CAD build for the part. Positions are in the model's coordinates, mm. A direction names the side the tool comes from. Round coordinates to 2 decimals unless told otherwise and drop trailing zeros. Loops run counter-clockwise (first coordinate to the right, second up) from the corner with the lowest first, then second, coordinate; pieces in that order, holes last. Notation, with made-up numbers: M 42.5,30 L 78.5,30 A24 cw 78.5,59 Z; hole C 8.5,33 d5. An arc over 180 degrees is marked long. Use one line per item in the form item = value.
Autodesk Inventor part; units mm, degrees
ref_plane "Work Plane1" through (0, 0, -15) normal (0, 0, 1) x (1, 0, 0)
ref_plane "YZ Plane" through (0, 0, 0) normal (1, 0, 0) x (0, 1, 0)
ref_plane "XZ Plane" through (0, 0, 0) normal (0, 1, 0) x (-1, 0, 0)
sketch "Sketch1" plane through (0, 0, 0) normal (0, 0, 1) x (1, 0, 0)
  line L0 (0, 0) -> (25, 0)
  line L1 (25, 0) -> (25, 40)
  line L2 (25, 40) -> (0, 40)
  line L3 (0, 40) -> (0, 0)
  dimension "d1" = 25
  dimension "d2" = 40
  dimension "d3" = 25
extrude "Extrusion1" add sketch "Sketch1" against normal blind 30
sketch "Sketch2" plane through (25, 0, 0) normal (1, 0, 0) x (0, 0, -1)
  line L0 (0, 0) -> (30, 0)
  circle A0 centre (15, 6.56) radius 2.46
extrude "Extrusion2" cut sketch "Sketch2" against normal blind 30
sketch "Sketch3" plane through (0, 0, 0) normal (-1, 0, 0) x (0, 0, 1)
  line L0 (0, 0) -> (-30, 0)
  line L1 (-25.05, 0) -> (-4.95, 0)
  line L2 (-4.95, 0) -> (-4.95, 33.12)
  line L3 (-4.95, 33.12) -> (-25.05, 33.12)
  line L4 (-25.05, 33.12) -> (-25.05, 0)
  dimension "d11" = 20.1
extrude "Extrusion3" cut sketch "Sketch3" against normal blind 20
sketch "Sketch4" plane through (0, 0, 0) normal (0, -1, 0) x (1, 0, 0)
  line L0 (20, -4.95) -> (20, -25.05)
  line L1 (20, -15) -> (25, -15)
  line L2 (25, 0) -> (25, -30)
  line L3 (20, -8.025) -> (25, -8.025)
  line L4 (25, -8.025) -> (25, -21.975)
  line L5 (25, -21.975) -> (20, -21.975)
  line L6 (20, -21.975) -> (20, -8.025)
  line L7 (20, -8.025) -> (25, -21.975) construction
  line L8 (25, -8.025) -> (20, -21.975) construction
  line L9 (25, -12.54) -> (25, -17.46)
  point P0 (0, 0)
  point P1 (22.5, -15)
  dimension "d14" = 13.95
extrude "Extrusion4" add sketch "Sketch4" along normal blind 15
sketch "Sketch5" plane through (20, 0, 0) normal (-1, 0, 0) x (0, 0, 1)
  circle A0 centre (-15, 6.56) radius 2.46
  circle A1 centre (-15, 6.56) radius 4.7025
  circle A2 centre (-15, 6.56) radius 2.46
  circle A3 centre (-15, 6.56) radius 2.46
  point P0 (0, 0)
  dimension "d17" = 9.405
extrude "Extrusion5" cut sketch "Sketch5" against normal blind 2.1
sketch "Sketch6" plane through (25, 0, 0) normal (1, 0, 0) x (0, 0, -1)
  circle A0 centre (15, 6.56) radius 4.7025
  line L0 (15, 6.56) -> (15, 23.56)
  circle A1 centre (15, 23.56) radius 2.46
  point P0 (0, 0)
  dimension "d20" = 17
  dimension "d21" = 4.92
extrude "Extrusion6" cut sketch "Sketch6" against normal blind 10 contours A1
sketch "Sketch7" plane through (20, 0, 0) normal (-1, 0, 0) x (0, 0, 1)
  circle A0 centre (-15, 23.56) radius 2.46
  circle A1 centre (-15, 23.56) radius 4.7025
  point P0 (0, 0)
  dimension "d24" = 9.405
extrude "Extrusion7" cut sketch "Sketch7" against normal blind 2.1
sketch "Sketch9" plane through (25, 0, 0) normal (1, 0, 0) x (0, 0, -1)
  circle A0 centre (15, 6.56) radius 2.46
  circle A1 centre (15, 6.56) radius 2.46
  circle A2 centre (15, 23.56) radius 2.46
  circle A3 centre (15, 23.56) radius 2.46
  line L0 (30, 40) -> (30, 0)
  line L1 (30, 0) -> (30, 40)
  line L2 (30, 40) -> (0, 40)
  line L3 (0, 40) -> (0, 0)
  line L4 (0, 0) -> (8.025, 0)
  line L5 (21.975, 0) -> (21.975, -15)
  line L6 (21.975, -15) -> (8.025, -15)
  line L7 (8.025, -15) -> (8.025, 0)
  line L8 (0, 0) -> (8.025, 0)
  line L9 (21.975, 0) -> (30, 0)
extrude "Extrusion8" add sketch "Sketch9" along normal blind 5
sketch "Sketch10" plane through (0, 40, 0) normal (0, 1, 0) x (1, 0, 0)
  line L0 (0, 30) -> (30, 30)
  line L1 (30, 0) -> (0, 0)
  line L2 (0, 30) -> (30, 30)
  line L3 (30, 30) -> (30, 0)
  line L4 (30, 0) -> (0, 0)
  line L5 (0, 0) -> (0, 30)
extrude "Extrusion9" add sketch "Sketch10" along normal blind 30
sketch "Sketch12" plane through (30, 0, 0) normal (1, 0, 0) x (0, 0, -1)
  circle A0 centre (15, 6.56) radius 2.46
  line L0 (15, 6.56) -> (15, 15.06)
  circle A1 centre (15, 15.06) radius 2.525
  point P0 (0, 0)
  dimension "d31" = 8.5
  dimension "d33" = 5.05
extrude "Extrusion10" cut sketch "Sketch12" against normal blind 30 contours A1
sketch "Sketch15" plane through (0, 0, -25.05) normal (-1, 0, 0) x (0, 0, 1)
  line L0 (0, 33.12) -> (20.1, 33.12)
  line L1 (20.1, 33.12) -> (20.1, 0)
  line L2 (0, 33.12) -> (20.1, 33.12)
  line L3 (20.1, 33.12) -> (20.1, 31.1)
  line L4 (20.1, 31.1) -> (0, 31.1)
  line L5 (0, 31.1) -> (0, 33.12)
  point P0 (25.05, 0)
  dimension "d57" = 2.02
extrude "Extrusion13" add sketch "Sketch15" against normal blind 20
sketch "Sketch17" plane through (0, 0, 0) normal (0, 0, 1) x (1, 0, 0)
  line L0 (0, 70) -> (30, 70)
  line L1 (30, 70) -> (50.0622, 90.0622)
  line L2 (30, 70) -> (80, 70) construction
  line L3 (11.9522, 97.2454) -> (0, 85.2932)
  line L4 (0, 70) -> (0, 85.2932)
  line L5 (0, 70) -> (0, 0)
  line L6 (0, 70) -> (30, 70)
  line L7 (10.923, 112.2849) -> (0, 120.567)
  line L8 (50.0622, 105.3553) -> (50.0622, 120.567)
  line L9 (50.0622, 105.3553) -> (50.0622, 90.0622)
  arc A0 (11.9522, 97.2454) -> (10.923, 112.2849) centre (4.8811, 104.3165) ccw
  line L10 (0, 144.567) -> (30, 144.567)
  line L11 (30, 144.567) -> (50.0622, 120.567)
  line L12 (4, 142.567) -> (0, 144.567)
  line L13 (4, 122.567) -> (0, 120.567)
  line L14 (4, 122.567) -> (8, 132.567)
  line L15 (8, 132.567) -> (4, 142.567)
  dimension "d61" = 45
  dimension "d62" = 32.0271
  dimension "d72" = 10
extrude "Extrusion14" add sketch "Sketch17" against normal blind 30
sketch "Sketch22" plane through (0, 0, 0) normal (0, 0, 1) x (1, 0, 0)
  line L0 (11.9522, 97.2454) -> (0, 85.2932)
  line L1 (0, 85.2932) -> (11.9522, 97.2454)
  arc A0 (11.9522, 97.2454) -> (10.923, 112.2849) centre (4.8811, 104.3165) ccw
  arc A1 (11.9522, 97.2454) -> (10.923, 112.2849) centre (4.8811, 104.3165) ccw
  line L2 (0, 120.567) -> (10.923, 112.2849)
  line L3 (10.923, 112.2849) -> (0, 120.567)
  line L4 (0, 120.567) -> (4, 122.567)
  line L5 (0, 120.567) -> (4, 122.567)
  line L6 (4, 122.567) -> (8, 132.567)
  line L7 (4, 122.567) -> (8, 132.567)
  line L8 (8, 132.567) -> (4, 142.567)
  line L9 (8, 132.567) -> (4, 142.567)
  line L10 (4, 142.567) -> (0, 144.567)
  line L11 (4, 142.567) -> (0, 144.567)
  line L12 (0, 144.567) -> (30, 144.567)
  line L13 (0, 144.567) -> (30, 144.567)
  line L14 (50.0622, 120.567) -> (30, 144.567)
  line L15 (30, 144.567) -> (50.0622, 120.567)
  line L16 (50.0622, 120.567) -> (50.0622, 90.0622)
  line L17 (50.0622, 120.567) -> (50.0622, 90.0622)
  line L18 (30, 70) -> (50.0622, 90.0622)
  line L19 (50.0622, 90.0622) -> (30, 70)
  line L20 (0, 0) -> (0, 85.2932)
  line L21 (0, 85.2932) -> (0, 55.2932)
  line L22 (0, 55.2932) -> (30, 55.2932)
  line L23 (30, 0) -> (30, 70)
  line L24 (30, 55.2932) -> (30, 70)
  dimension "d83" = 30
extrude "Extrusion15" add sketch "Sketch22" along normal blind 45
ref_plane "Work Plane1" through (0, 0, -15) normal (0, 0, 1) x (1, 0, 0)
mirror "Mirror1" about plane through (0, 0, -15) normal (0, 0, 1) of "Extrusion15"
properties part number "rec_c_20mm_x_120mm"
1. Cut at B-B on z = 7.5. Write the cut outline in (x, y), and give its area (3 significant figures).
Completed:
outline = M 0,55.29 L 30,55.29 L 30,70 L 50.06,90.06 L 50.06,120.57 L 30,144.57 L 0,144.57 L 4,142.57 L 8,132.57 L 4,122.57 L 0,120.57 L 10.92,112.28 A10 cw 11.95,97.25 L 0,85.29 Z
area = 3,280 mm2
2. Cut at D-D on y = 65. Write the cut outline in (x, z), and give its area (3 significant figures).
Completed:
outline = M 0,-75 L 30,-75 L 30,45 L 0,45 Z
area = 3,600 mm2
3. Drop flat-ended pins along their axis: P1, Ø12, axis at x = 38, z = -30, coming from the +Y side; P2, Ø11, axis at x = 24, y = -10, coming from the -Z side (3 decimals); P3, Ø10, axis at y = 62.5, z = -14, coming from the +X side. Give the stop position or say it passes through.
Completed:
P1 = 142.17
P2 = -21.975
P3 = 30
4. Cut at A-A on y = 23.56. Write the cut outline in (x, z).
Completed:
outline = M 0,-30 L 30,-30 L 30,-17.46 L 22.1,-17.46 L 22.1,-19.7 L 20,-19.7 L 20,-25.05 L 0,-25.05 Z; M 0,-4.95 L 20,-4.95 L 20,-10.3 L 22.1,-10.3 L 22.1,-12.54 L 30,-12.54 L 30,0 L 0,0 Z
5. Tool access for faces 1 (the face through (22.1, 21.5, -13)), 2 (the face through (15, 28, -30)), 3 (the face through (15, 28, 0)): list every direction of +Z, -Z, +X, -X, +Y, -Y with a clear straight run to the whole face (end or side of a thin tool).
Completed:
face_1 = -X
face_2 = -Z, +X, -X, -Y
face_3 = +Z, +X, -X, -Y
6. Cut at C-C on z = -15. State how many separate pieces and enclosed holes the cut face has, and give its area (3 significant figures).
Completed:
separate_pieces = 4
enclosed_holes = 0
area = 4,300 mm2
7. Probe line 1 along Y through (x, z) = (27, -15) (3 decimals); line 2 along Y through (x, z) = (21.75, -15) (1 decimal); line 3 along Z through (x, y) = (27, 15.06) (3 decimals). List the from-to ranges inside material, lowest first. Write a range as from..to.
Completed:
line_1 = -15..4.1, 9.02..12.535, 17.585..21.1, 26.02..144.567
line_2 = -15..1.9, 11.3..12.5, 17.6..18.9, 28.3..144.6
line_3 = -30..-17.525, -12.475..0
8. Pull direction Z, two halves, no side cores. Call faces 4 (the face through (25, 101, 45)), 5 (the face through (2.03, 121.58, -14.16)), 6 (the face through (25.995, 7.502, -17.272)): +Z half, -Z half, draft (parallel to the pull), parting line (faces both ways), or undercut.
Completed:
face_4 = +Z half
face_5 = draft
face_6 = undercut
